from build123d import *

# Parameters (mm, degrees)
SKETCH_1_R      = 28
SKETCH_1_R_2    = 2.08
SKETCH_1_R_3    = 8.75
SKETCH_1_R_4    = 1.25
SKETCH_1_R_5    = 1.5
EXTRUDE_1_DEPTH = 2


with BuildPart() as part:
    # 草图1 → 凸台-拉伸1 (new body)
    with BuildSketch(Plane.XY):
        Circle(SKETCH_1_R)
        with Locations((-13.53, 0)):
            Circle(SKETCH_1_R_2, mode=Mode.SUBTRACT)
        with Locations((6.765, 11.717323713)):
            Circle(SKETCH_1_R_2, mode=Mode.SUBTRACT)
        with Locations((6.765, -11.717323713)):
            Circle(SKETCH_1_R_2, mode=Mode.SUBTRACT)
        Circle(SKETCH_1_R_3, mode=Mode.SUBTRACT)
        with Locations((12.351862398, 21.735489304)):
            Circle(SKETCH_1_R_4, mode=Mode.SUBTRACT)
        with Locations((24.9994171, 0.170718032)):
            Circle(SKETCH_1_R_4, mode=Mode.SUBTRACT)
        with Locations((12.647554702, -21.564771273)):
            Circle(SKETCH_1_R_4, mode=Mode.SUBTRACT)
        with Locations((-12.351862398, -21.735489304)):
            Circle(SKETCH_1_R_4, mode=Mode.SUBTRACT)
        with Locations((-24.9994171, -0.170718032)):
            Circle(SKETCH_1_R_4, mode=Mode.SUBTRACT)
        with Locations((-12.647554702, 21.564771273)):
            Circle(SKETCH_1_R_4, mode=Mode.SUBTRACT)
        with Locations((-7.411117439, -13.041293583)):
            Circle(SKETCH_1_R_5, mode=Mode.SUBTRACT)
        with Locations((-7.588532821, 12.938862764)):
            Circle(SKETCH_1_R_5, mode=Mode.SUBTRACT)
        with Locations((14.99965026, 0.102430819)):
            Circle(SKETCH_1_R_5, mode=Mode.SUBTRACT)
    extrude(amount=EXTRUDE_1_DEPTH)


solid = part.part
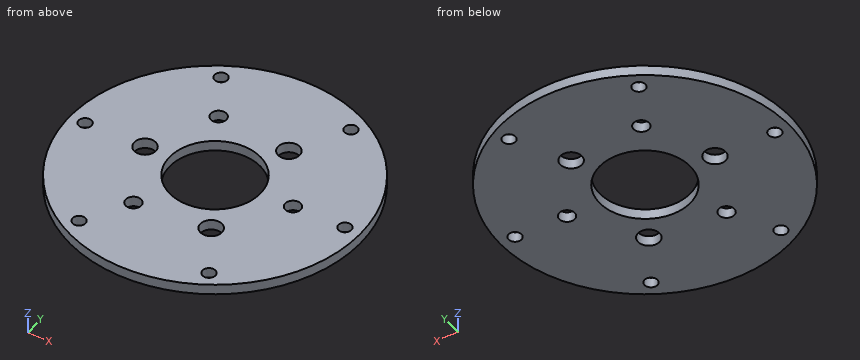
Design review of the part built by this model. Coordinates are the model's own, in mm. Round coordinates to 2 decimals unless told otherwise and drop trailing zeros. Write each loop counter-clockwise with the first axis right and the second up, starting at its lowest first coordinate (ties: lowest second). Pieces come first, ordered by that corner, then holes. Notation, with made-up numbers: (-28.75, 47.5) - (-11.75, 47.5) arc R19 ccw to (-11.75, 63.5) - close; hole circle Ø1 at (60.5, 6). An arc over 180 degrees is marked (long way). Return JSON: item names as keys, results as strings. Group by question number.
Item 1: For probe 1 along X at (y, z) = (22, 1.75); probe 2 along Y at (x, z) = (-13, 1.65); probe 3 along X at (y, z) = (-10, 1.6), list the stretches that pass through material, from the lowest coordinate up. Write a range as [from, to].
Item 2: We need section D-D on y = -18. Write out the cut boundary in (x, z), and give its area (3 significant figures).
Item 3: Insertion check: P1, Ø1, axis at y = 16, z = 1.5, coming from the +X side. The pin has a flat end and moves straight along its axis. Give the tip position at first contact, or say it passes through.
Item 4: We need section B-B on y = 3. Write out the cut boundary in (x, z).
Item 5: We need section C-C on z = 1.2. Give the number of separate pieces and of enclosed holes in the cut face, and give its area (3 significant figures).
Item 6: We need section A-A on x = 0. Write out the cut boundary in (y, z).
Model answer:
{
 "1": {"probe 1": "x = [-17.32, -13.82], [-11.48, 11.13], [13.57, 17.32]", "probe 2": "y = [-24.8, -22.8], [-20.67, -2.01], [2.01, 20.37], [22.76, 24.8]", "probe 3": "x = [-26.15, 5.59], [7.94, 26.15]"},
 "2": {"outline": "(-21.45, 0) - (21.45, 0) - (21.45, 2) - (-21.45, 2) - close", "area": "85.8 mm²"},
 "3": {"P1": "stops at x = 23.32"},
 "4": {"outline": "(-27.84, 0) - (-8.22, 0) - (-8.22, 2) - (-27.84, 2) - close; (8.22, 0) - (27.84, 0) - (27.84, 2) - (8.22, 2) - close"},
 "5": {"separate pieces": "1", "enclosed holes": "13", "area": "2,130 mm²"},
 "6": {"outline": "(-28, 0) - (-8.75, 0) - (-8.75, 2) - (-28, 2) - close; (8.75, 0) - (28, 0) - (28, 2) - (8.75, 2) - close"}
}
